from build123d import *

# Parameters (mm, degrees)
BOSS_EXTRUDE1_DEPTH = 3
CUT_EXTRUDE1_REACH  = 77.661
SKETCH1_3_R         = 1.25
BOSS_EXTRUDE2_START = 8.86
BOSS_EXTRUDE2_DEPTH = 8.86
BOSS_EXTRUDE3_START = 1.5
SKETCH1_5_R         = 3.21
SKETCH1_5_R_2       = 1.25
BOSS_EXTRUDE3_DEPTH = 1.5
SKETCH2_W           = 12.28
SKETCH2_H           = 8.73
CUT_EXTRUDE2_DEPTH  = 3
SKETCH5_R           = 1.95
BOSS_EXTRUDE5_DEPTH = 3


with BuildPart() as part:
    # Sketch1 → Boss-Extrude1 (new body)
    with BuildSketch(Plane(origin=(0, 0, 0), x_dir=(1, 0, 0), z_dir=(0, 1, 0))):
        with BuildLine():
            Line((3.81, 3), (49.09, 3))
            ThreePointArc((49.09, 3), (53.90539718, 1.00539718), (55.9, -3.81))
            Line((55.9, -3.81), (55.9, -44.09))
            ThreePointArc((55.9, -44.09), (53.90539718, -48.90539718), (49.09, -50.9))
            Line((49.09, -50.9), (3.81, -50.9))
            ThreePointArc((3.81, -50.9), (-1.00539718, -48.90539718), (-3, -44.09))
            Line((-3, -44.09), (-3, -3.81))
            ThreePointArc((-3, -3.81), (-1.00539718, 1.00539718), (3.81, 3))
        make_face()
    extrude(amount=-BOSS_EXTRUDE1_DEPTH)

    # Sketch1_3 → Cut-Extrude1 (cut, up to next)
    with BuildSketch(Plane(origin=(0, 0, 0), x_dir=(1, 0, 0), z_dir=(0, 1, 0)), mode=Mode.PRIVATE) as cut_extrude1_sk1:
        with Locations(Location((3.81, -3.81, 0), (0, 0, 270))):
            Circle(SKETCH1_3_R)
    cut_extrude1_tool1 = extrude(cut_extrude1_sk1.sketch, amount=-CUT_EXTRUDE1_REACH, mode=Mode.PRIVATE) & part.part
    # Sketch1_3 → Cut-Extrude1 (cut, up to next)
    with BuildSketch(Plane(origin=(0, 0, 0), x_dir=(1, 0, 0), z_dir=(0, 1, 0)), mode=Mode.PRIVATE) as cut_extrude1_sk2:
        with Locations(Location((3.81, -44.09, 0), (0, 0, 270))):
            Circle(SKETCH1_3_R)
    cut_extrude1_tool2 = extrude(cut_extrude1_sk2.sketch, amount=-CUT_EXTRUDE1_REACH, mode=Mode.PRIVATE) & part.part
    # Sketch1_3 → Cut-Extrude1 (cut, up to next)
    with BuildSketch(Plane(origin=(0, 0, 0), x_dir=(1, 0, 0), z_dir=(0, 1, 0)), mode=Mode.PRIVATE) as cut_extrude1_sk3:
        with Locations(Location((49.09, -44.09, 0), (0, 0, 270))):
            Circle(SKETCH1_3_R)
    cut_extrude1_tool3 = extrude(cut_extrude1_sk3.sketch, amount=-CUT_EXTRUDE1_REACH, mode=Mode.PRIVATE) & part.part
    # Sketch1_3 → Cut-Extrude1 (cut, up to next)
    with BuildSketch(Plane(origin=(0, 0, 0), x_dir=(1, 0, 0), z_dir=(0, 1, 0)), mode=Mode.PRIVATE) as cut_extrude1_sk4:
        with Locations(Location((49.09, -3.81, 0), (0, 0, 270))):
            Circle(SKETCH1_3_R)
    cut_extrude1_tool4 = extrude(cut_extrude1_sk4.sketch, amount=-CUT_EXTRUDE1_REACH, mode=Mode.PRIVATE) & part.part
    add(cut_extrude1_tool1.solids().sort_by_distance((3.81, 0, 3.81))[0], mode=Mode.SUBTRACT)
    add(cut_extrude1_tool2.solids().sort_by_distance((3.81, 0, 44.09))[0], mode=Mode.SUBTRACT)
    add(cut_extrude1_tool3.solids().sort_by_distance((49.09, 0, 44.09))[0], mode=Mode.SUBTRACT)
    add(cut_extrude1_tool4.solids().sort_by_distance((49.09, 0, 3.81))[0], mode=Mode.SUBTRACT)

    # Sketch1_4 → Boss-Extrude2 (add)
    with BuildSketch(Plane(origin=(0, 0, 0), x_dir=(1, 0, 0), z_dir=(0, 1, 0)).offset(BOSS_EXTRUDE2_START)):
        with BuildLine():
            ThreePointArc((-3, -3.81), (-1.00539718, 1.00539718), (3.81, 3))
            Line((3.81, 3), (49.09, 3))
            ThreePointArc((49.09, 3), (53.90539718, 1.00539718), (55.9, -3.81))
            Line((55.9, -3.81), (55.9, -44.09))
            ThreePointArc((55.9, -44.09), (53.90539718, -48.90539718), (49.09, -50.9))
            Line((49.09, -50.9), (3.81, -50.9))
            ThreePointArc((3.81, -50.9), (-1.00539718, -48.90539718), (-3, -44.09))
            Line((-3, -44.09), (-3, -3.81))
        make_face()
        with BuildLine():
            Line((52.9, -3.81), (52.9, -44.09))
            ThreePointArc((52.9, -44.09), (51.784076836, -46.784076836), (49.09, -47.9))
            Line((49.09, -47.9), (3.81, -47.9))
            ThreePointArc((3.81, -47.9), (1.115923164, -46.784076836), (0, -44.09))
            Line((0, -44.09), (0, -3.81))
            ThreePointArc((0, -3.81), (1.115923164, -1.115923164), (3.81, 0))
            Line((3.81, 0), (49.09, 0))
            ThreePointArc((49.09, 0), (51.784076836, -1.115923164), (52.9, -3.81))
        make_face(mode=Mode.SUBTRACT)
    extrude(amount=-BOSS_EXTRUDE2_DEPTH)

    # Sketch1_5 → Boss-Extrude3 (add)
    # profile 1 of 4: a face of its own
    with BuildSketch(Plane(origin=(0, 0, 0), x_dir=(1, 0, 0), z_dir=(0, 1, 0)).offset(BOSS_EXTRUDE3_START)):
        with Locations(Location((49.09, -3.81, 0), (0, 0, 90))):
            Circle(SKETCH1_5_R)
        with Locations(Location((49.09, -3.81, 0), (0, 0, 270))):
            Circle(SKETCH1_5_R_2, mode=Mode.SUBTRACT)
    # profile 2 of 4: a face of its own
    with BuildSketch(Plane(origin=(0, 0, 0), x_dir=(1, 0, 0), z_dir=(0, 1, 0)).offset(BOSS_EXTRUDE3_START)):
        with Locations(Location((49.09, -44.09, 0), (0, 0, 90))):
            Circle(SKETCH1_5_R)
        with Locations(Location((49.09, -44.09, 0), (0, 0, 270))):
            Circle(SKETCH1_5_R_2, mode=Mode.SUBTRACT)
    # profile 3 of 4: a face of its own
    with BuildSketch(Plane(origin=(0, 0, 0), x_dir=(1, 0, 0), z_dir=(0, 1, 0)).offset(BOSS_EXTRUDE3_START)):
        with Locations(Location((3.81, -44.09, 0), (0, 0, 90))):
            Circle(SKETCH1_5_R)
        with Locations(Location((3.81, -44.09, 0), (0, 0, 270))):
            Circle(SKETCH1_5_R_2, mode=Mode.SUBTRACT)
    # profile 4 of 4: a face of its own
    with BuildSketch(Plane(origin=(0, 0, 0), x_dir=(1, 0, 0), z_dir=(0, 1, 0)).offset(BOSS_EXTRUDE3_START)):
        with Locations(Location((3.81, -3.81, 0), (0, 0, 90))):
            Circle(SKETCH1_5_R)
        with Locations(Location((3.81, -3.81, 0), (0, 0, 270))):
            Circle(SKETCH1_5_R_2, mode=Mode.SUBTRACT)
    extrude(amount=-BOSS_EXTRUDE3_DEPTH)

    # Sketch2 → Cut-Extrude2 (cut)
    with BuildSketch(Plane.XY.offset(50.9)):
        with Locations((18.5, 4.5)):
            Rectangle(SKETCH2_W, SKETCH2_H)
    extrude(amount=-CUT_EXTRUDE2_DEPTH, mode=Mode.SUBTRACT)

    # Sketch5 → Boss-Extrude5 (add)
    with BuildSketch(Plane(origin=(0, 0, -3), x_dir=(-1, 0, 0), z_dir=(0, 0, -1))):
        with BuildLine():
            Line((-31.45, 8.86), (-21.45, 8.86))
            Line((-21.45, 8.86), (-21.45, 14.96))
            ThreePointArc((-21.45, 14.96), (-22.592283553, 17.717716447), (-25.35, 18.86))
            Line((-25.35, 18.86), (-27.55, 18.86))
            ThreePointArc((-27.55, 18.86), (-30.307716447, 17.717716447), (-31.45, 14.96))
            Line((-31.45, 14.96), (-31.45, 8.86))
        make_face()
        with Locations((-26.45, 13.86)):
            Circle(SKETCH5_R, mode=Mode.SUBTRACT)
    extrude(amount=-BOSS_EXTRUDE5_DEPTH)


solid = part.part
Could you check a few things on this model? Use its own coordinates, in mm. A direction names the side the tool comes from. Coordinates: 2 decimals unless noted, no trailing zeros. Order: outer loops, then holes, each group sorted by start corner. A loop starts at its lowest first (then second) coordinate and runs counter-clockwise, first axis right, second up.
Q1. Please list where these lines run through material, in increasing order: L1, parallel to X at y = -0.6, z = 3.81; L2, parallel to X at y = 2, z = 42; L3, parallel to Y at x = 24, z = 19.5.
Q2. Will these pins go through, and if not, where does the flat tip stop? pin 1 (7 mm diameter, centred on x = 48.5, z = 44, fed in from +Y); pin 2 (25 mm diameter, centred on x = 36.5, z = 14.5, fed in from +Y); pin 3 (1.5 mm diameter, centred on y = 6.5, z = 49.5, fed in from -X).
Q3. Suppose I cut it at D-D on x = 11.5. Please give me the cut outline in (y, z), and give its area (3 significant figures).
Q4. Suppose I cut it at C-C on y = 5. Please give me the cut outline in (x, z), and give its area (3 significant figures).
Q5. Which directions (+Z, -Z, +X, -X, +Y, -Y) give clear straight access to the entire face, cutting with the end or side of a thin tool? Please do faces 4 (the flat face through (31.45, 12, -2)), 5 (the flat face through (18, 0.135, 49)), 6 (the cylindrical face through (45.907, 0.76, 44.508)).
Q6. Thinking about a two-plate mould opening in X: for faces 1 (the cylindrical face through (1.146, 4.492, 46.814)), 2 (the flat face through (26, 18.86, -2)), 3 (the cylindrical face through (53.96, 3.01, 48.85)), which applies, released by +X, released by -X, zero draft, split by the parting line, or undercut?
Q7. Suppose I cut it at B-B on z = 13.5. Please give me the cut outline in (x, y).
Q8. Suppose I cut it at A-A on x = 26.45. Please give me the cut outline in (y, z), and give its area (3 significant figures).
Answer:
1. L1: x = -3 to 2.56, 5.06 to 47.84, 50.34 to 55.9
1. L2: x = -3 to 0, 52.9 to 55.9
1. L3: y = -3 to 0
2. pin 1: stops at y = 1.5
2. pin 2: stops at y = 0
2. pin 3: stops at x = -1.16
3. outline: (-3, -3) - (8.86, -3) - (8.86, 0) - (0, 0) - (0, 47.9) - (8.86, 47.9) - (8.86, 50.9) - (-3, 50.9) - close
3. area: 215 mm2
4. outline: (-3, 3.81) arc R6.81 ccw to (3.81, -3) - (49.09, -3) arc R6.81 ccw to (55.9, 3.81) - (55.9, 44.09) arc R6.81 ccw to (49.09, 50.9) - (24.64, 50.9) - (24.64, 47.9) - (49.09, 47.9) arc R3.81 cw to (52.9, 44.09) - (52.9, 3.81) arc R3.81 cw to (49.09, 0) - (3.81, 0) arc R3.81 cw to (0, 3.81) - (0, 44.09) arc R3.81 cw to (3.81, 47.9) - (12.36, 47.9) - (12.36, 50.9) - (3.81, 50.9) arc R6.81 ccw to (-3, 44.09) - close
4. area: 577 mm2
5. face 4: +Z, -Z, +X, +Y
5. face 5: +Z, +Y
5. face 6: +Y
6. face 1: undercut
6. face 2: zero draft
6. face 3: released by +X
7. outline: (-3, -3) - (55.9, -3) - (55.9, 8.86) - (52.9, 8.86) - (52.9, 0) - (0, 0) - (0, 8.86) - (-3, 8.86) - close
8. outline: (-3, -3) - (11.91, -3) - (11.91, 0) - (0, 0) - (0, 47.9) - (8.86, 47.9) - (8.86, 50.9) - (-3, 50.9) - close; (15.81, -3) - (18.86, -3) - (18.86, 0) - (15.81, 0) - close
8. area: 233 mm2
